Geometry: final body of the model. Coordinates: model frame, mm. Face numbers are marked on the shaded views. A direction names the side the tool comes from. Coordinates: 2 decimals unless noted, no trailing zeros. Write each loop counter-clockwise with the first axis right and the second up, starting at its lowest first coordinate (ties: lowest second). Pieces come first, ordered by that corner, then holes. Notation, with made-up numbers: (-28.75, 47.5) - (3.25, 47.5) arc R14 cw to (3.25, 68.5) - close; hole circle Ø1 at (-10, -12.75). An arc over 180 degrees is marked (long way). Answer as a JSON object with one key per item and string values. Group by question number.
Item 1: Section B-B on x = -26.5. Return loops of the section in (y, z), and give its area (3 significant figures).
Item 2: Set-up query: the marked faces 1 and 2. Return all of +Z, -Z, +X, -X, +Y, -Y with unobstructed straight access to the full face (end or side cutting, diameter ignored); none if empty.
Item 3: Line query: line 1 along Z through (x, y) = (28.5, -10.5); line 2 along Z through (x, y) = (23.5, -8.75); line 3 along Z through (x, y) = (18, -8). Output: solid intervals per line, ascending. Write a range as from..to.
Item 4: Section A-A on x = 0. Return loops of the section in (y, z), and give its area (3 significant figures).
Item 5: Section D-D on x = 24.5. Return loops of the section in (y, z), and give its area (3 significant figures).
Item 6: Section C-C on y = -10.5. Return loops of the section in (x, z), and give its area (3 significant figures).
Item 7: Mould query, pull axis X, two halves, no side actions, for the marked faces 3, 4 and 5. Classes: pulls with the +X half, pulls with the -X half, needs draft (parallel to the pull), parting line crosses it, or undercut.
Item 8: First-contact query: pin 1 Ø2 at (y, z) = (-11, -55.5) entering from +X; pin 2 Ø22 at (x, z) = (-8.5, 15) entering from +Y; pin 3 Ø1 at (y, z) = (-11, -70) entering from -X; pin 4 Ø3 at (y, z) = (-10.5, -85.6) entering from -X. Flat tips, straight axial feed; report the tip coordinate or a pass-through.
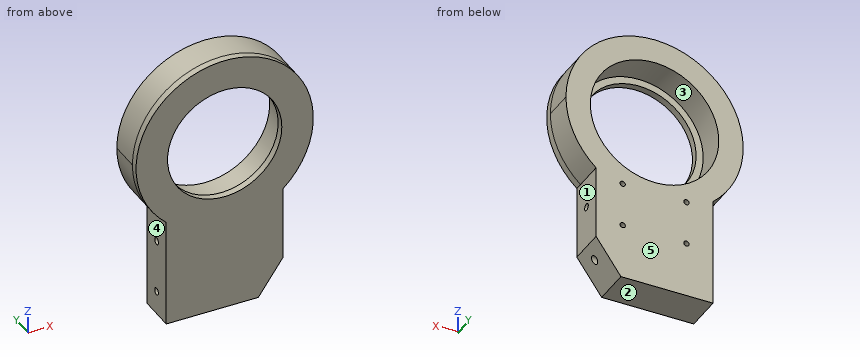
```python
from build123d import *

# Parameters (mm, degrees)
F0_R      = 36.25
F1_DEPTH  = 17
F2_R      = 32.25
F3_DEPTH  = 4
F4_R      = 1.5
F5_DEPTH  = 15
F8_DEPTH  = 25
F11_DEPTH = 25


with BuildPart() as f1:
    # F0 (on Front) → F1 (new body)
    with BuildSketch(Plane.XZ):
        with BuildLine():
            ThreePointArc((33, -37.56328), (45.552168, -20.615528), (50, 0))
            ThreePointArc((50, 0), (0, 50), (-50, 0))
            ThreePointArc((-50, 0), (-45.552168, -20.615528), (-33, -37.56328))
            Line((-33, -37.56328), (-33, -79))
            Line((-33, -79), (-33, -99))
            Line((-33, -99), (-18.995849, -99))
            Line((-18.995849, -99), (0, -99))
            Line((0, -99), (18.995849, -99))
            Line((18.995849, -99), (33, -79))
            Line((33, -79), (33, -37.56328))
        make_face()
        Circle(F0_R, mode=Mode.SUBTRACT)
    extrude(amount=F1_DEPTH)

    # F2 (on face) → F3 (join)
    with BuildSketch(Plane.XZ.offset(17)):
        with BuildLine():
            Line((33, -79), (33, -37.56328))
            ThreePointArc((33, -37.56328), (0, 50), (-33, -37.56328))
            Line((-33, -37.56328), (-33, -99))
            Line((-33, -99), (18.995849, -99))
            Line((18.995849, -99), (33, -79))
        make_face()
        Circle(F2_R, mode=Mode.SUBTRACT)
    extrude(amount=F3_DEPTH)

    # F4 (on face) → F5 (cut)
    with BuildSketch(Plane(origin=(0, 0, 0), x_dir=(-1, 0, 0), z_dir=(0, 1, 0))):
        with Locations((-18, -42.60355)):
            Circle(F4_R)
        with Locations((18, -42.60355)):
            Circle(F4_R)
        with Locations((18, -67.60355)):
            Circle(F4_R)
        with Locations((-18, -67.60355)):
            Circle(F4_R)
    extrude(amount=-F5_DEPTH, mode=Mode.SUBTRACT)

    # F7 (on offset) → F8 (cut)
    with BuildSketch(Plane.YZ.offset(21)):
        with BuildLine():
            ThreePointArc((-12.5, -85.60355), (-10.5, -87.60355), (-8.5, -85.60355))
            Line((-8.5, -85.60355), (-12.5, -85.60355))
        make_face()
        with BuildLine():
            Line((-12.5, -85.60355), (-8.5, -85.60355))
            ThreePointArc((-8.5, -85.60355), (-10.5, -83.60355), (-12.5, -85.60355))
        make_face()
        with BuildLine():
            ThreePointArc((-12.5, -55.10355), (-10.5, -57.10355), (-8.5, -55.10355))
            Line((-8.5, -55.10355), (-12.5, -55.10355))
        make_face()
        with BuildLine():
            Line((-12.5, -55.10355), (-8.5, -55.10355))
            ThreePointArc((-8.5, -55.10355), (-10.5, -53.10355), (-12.5, -55.10355))
        make_face()
    extrude(amount=F8_DEPTH, mode=Mode.SUBTRACT)

    # F10 (on offset) → F11 (cut)
    with BuildSketch(Plane.YZ.offset(-21)):
        with BuildLine():
            ThreePointArc((-12.5, -85.60355), (-10.5, -87.60355), (-8.5, -85.60355))
            Line((-8.5, -85.60355), (-12.5, -85.60355))
        make_face()
        with BuildLine():
            Line((-12.5, -85.60355), (-8.5, -85.60355))
            ThreePointArc((-8.5, -85.60355), (-10.5, -83.60355), (-12.5, -85.60355))
        make_face()
        with BuildLine():
            ThreePointArc((-12.5, -55.10355), (-10.5, -57.10355), (-8.5, -55.10355))
            Line((-8.5, -55.10355), (-12.5, -55.10355))
        make_face()
        with BuildLine():
            Line((-12.5, -55.10355), (-8.5, -55.10355))
            ThreePointArc((-8.5, -55.10355), (-10.5, -53.10355), (-12.5, -55.10355))
        make_face()
    extrude(amount=-F11_DEPTH, mode=Mode.SUBTRACT)


solid = f1.part
```
Checks:
{
 "1": {"outline": "(-21, -99) - (0, -99) - (0, -24.73) - (-17, -24.73) - (-17, -18.38) - (-21, -18.38) - close; (-21, 18.38) - (-17, 18.38) - (-17, 24.73) - (0, 24.73) - (0, 42.4) - (-21, 42.4) - close; hole circle Ø4 at (-10.5, -85.6); hole circle Ø4 at (-10.5, -55.1)", "area": "1,960 mm^2"},
 "2": {"face 1": "-Z, +X, +Y, -Y", "face 2": "-Z, +X, -X, +Y, -Y"},
 "3": {"line 1": "-83.6..-57.1, -53.1..-22.4, 22.4..41.08", "line 2": "-92.57..-86.57, -84.64..-56.07, -54.14..-27.6, 27.6..44.13", "line 3": "-99..-69.1, -66.1..-44.1, -41.1..-31.47, 31.47..46.65"},
 "4": {"outline": "(-21, -99) - (0, -99) - (0, -36.25) - (-17, -36.25) - (-17, -32.25) - (-21, -32.25) - close; (-21, 32.25) - (-17, 32.25) - (-17, 36.25) - (0, 36.25) - (0, 50) - (-21, 50) - close", "area": "1,640 mm^2"},
 "5": {"outline": "(-21, -91.14) - (0, -91.14) - (0, -26.72) - (-17, -26.72) - (-17, -20.97) - (-21, -20.97) - close; (-21, 20.97) - (-17, 20.97) - (-17, 26.72) - (0, 26.72) - (0, 43.59) - (-21, 43.59) - close; hole circle Ø4 at (-10.5, -85.6); hole circle Ø4 at (-10.5, -55.1)", "area": "1,730 mm^2"},
 "6": {"outline": "(-33, -99) - (19, -99) - (26.98, -87.6) - (21, -87.6) - (21, -83.6) - (29.78, -83.6) - (33, -79) - (33, -57.1) - (21, -57.1) - (21, -53.1) - (33, -53.1) - (33, -37.56) arc R50 ccw (long way) to (-33, -37.56) - (-33, -53.1) - (-21, -53.1) - (-21, -57.1) - (-33, -57.1) - (-33, -83.6) - (-21, -83.6) - (-21, -87.6) - (-33, -87.6) - close; hole circle Ø72.5 at (0, 0); hole circle Ø3 at (-18, -67.6); hole circle Ø3 at (-18, -42.6); hole circle Ø3 at (18, -67.6); hole circle Ø3 at (18, -42.6)", "area": "6,880 mm^2"},
 "7": {"face 3": "undercut", "face 4": "pulls with the -X half", "face 5": "needs draft"},
 "8": {"pin 1": "x = 21", "pin 2": "through", "pin 3": "x = -33", "pin 4": "x = -21"}
}
